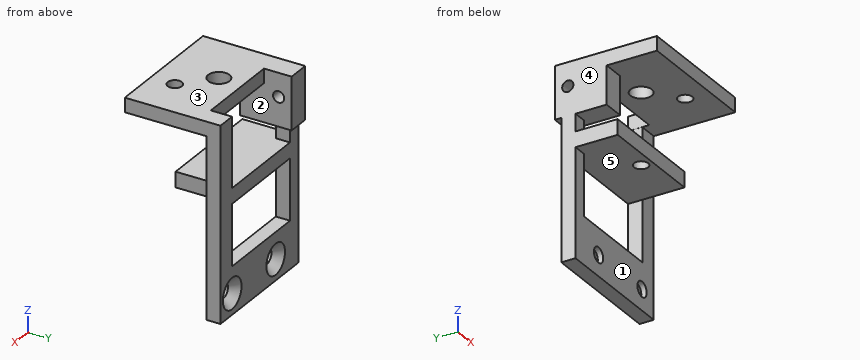
from build123d import *

# Parameters (mm, degrees)
SKETCH1_R                                        = 3.175
SKETCH1_R_2                                      = 4.762499999
BOSS_EXTRUDE1_DEPTH                              = 6.35
BOSS_EXTRUDE2_DEPTH                              = 23.368
SKETCH3_W                                        = 6.35
SKETCH3_H                                        = 78.34
SKETCH3_W_2                                      = 8.382
BOSS_EXTRUDE3_DEPTH                              = 6.35
CUT_EXTRUDE1_REACH                               = 104.101
SKETCH4_R                                        = 2.5
BOSS_EXTRUDE4_DEPTH                              = 6.35
CSK_FOR_1_4_FLAT_HEAD_MACHINE_SCREW1_D           = 6.7564
CSK_FOR_1_4_FLAT_HEAD_MACHINE_SCREW1_CSINK_D     = 13.6398
CSK_FOR_1_4_FLAT_HEAD_MACHINE_SCREW1_CSINK_ANGLE = 82
SKETCH8_W                                        = 48.768
SKETCH8_H                                        = 6.843039895
BOSS_EXTRUDE5_DEPTH                              = 25.146
CUT_EXTRUDE2_REACH                               = 68.059
SKETCH10_R                                       = 3.175


with BuildPart() as part:
    # Sketch1 → Boss-Extrude1 (new body)
    with BuildSketch(Plane.XY):
        Polygon((23.52260518, 29.069744957), (31.942128684, 29.069744957), (31.942128684, -13.602255043), (-25.207871316, -13.602255043), (-25.207871316, 8.844196721), (-25.207871316, 31.958196721), (-18.857871316, 31.958196721), (-15.310946905, 31.958196721), (-15.310946905, 22.656471706), (-15.310946905, 19.620299994), (23.52260518, 19.620299994), (23.52260518, 22.656471706), align=None)
        with Locations((12.892128684, -2.934255043)):
            Circle(SKETCH1_R, mode=Mode.SUBTRACT)
        with Locations((6.7e-08, 8.844196721)):
            Circle(SKETCH1_R_2, mode=Mode.SUBTRACT)
    extrude(amount=-BOSS_EXTRUDE1_DEPTH)

    # Sketch2 → Boss-Extrude2 (add)
    with BuildSketch(Plane.XY):
        Polygon((-15.310946905, 31.958196721), (-18.857871316, 31.958196721), (-25.207871316, 31.958196721), (-25.207871316, 8.844196721), (-18.857871316, 8.844196721), (-15.310946905, 8.844196721), (-15.310946905, 19.620299994), align=None)
    extrude(amount=-BOSS_EXTRUDE2_DEPTH)

    # Sketch3 → Boss-Extrude3 (add)
    with BuildSketch(Plane(origin=(0, 29.069744957, 0), x_dir=(1, 0, 0), z_dir=(0, 1, 0))):
        with Locations((-22.032871316, 39.17)):
            Rectangle(SKETCH3_W, SKETCH3_H)
        with Locations((27.751128684, 39.17)):
            Rectangle(SKETCH3_W_2, SKETCH3_H)
    extrude(amount=-BOSS_EXTRUDE3_DEPTH)

    # Sketch4 → Cut-Extrude1 (cut, up to next)
    with BuildSketch(Plane.ZY.offset(25.207871316), mode=Mode.PRIVATE) as cut_extrude1_sk1:
        with Locations(Location((-10.437499124, 26.162307082, 0), (0, 0, 270))):
            Circle(SKETCH4_R)
    cut_extrude1_tool1 = extrude(cut_extrude1_sk1.sketch, amount=-CUT_EXTRUDE1_REACH, mode=Mode.PRIVATE) & part.part
    add(cut_extrude1_tool1.solids().sort_by_distance((-25.207871, 26.162307, -10.437499))[0], mode=Mode.SUBTRACT)

    # Sketch5 → Boss-Extrude4 (add)
    with BuildSketch(Plane(origin=(0, 29.069744957, 0), x_dir=(1, 0, 0), z_dir=(0, 1, 0))):
        Polygon((-25.207871316, 78.34), (-25.207871316, 65.022649662), (31.942128684, 65.022649662), (31.942128684, 78.34), (31.942128684, 86.081334737), (-25.207871316, 86.081334737), align=None)
    extrude(amount=-BOSS_EXTRUDE4_DEPTH)

    # CSK for 1/4 Flat Head Machine Screw1 (through all)
    with Locations(Plane(origin=(0, 29.069744957, 0), x_dir=(1, 0, 0), z_dir=(0, 1, 0))):
        with Locations((-8.384740386, 76.819020678), (23.394249394, 76.819020678)):
            CounterSinkHole(CSK_FOR_1_4_FLAT_HEAD_MACHINE_SCREW1_D / 2, CSK_FOR_1_4_FLAT_HEAD_MACHINE_SCREW1_CSINK_D / 2, counter_sink_angle=CSK_FOR_1_4_FLAT_HEAD_MACHINE_SCREW1_CSINK_ANGLE)

    # Sketch8 → Boss-Extrude5 (add)
    with BuildSketch(Plane(origin=(0, 29.069744957, 0), x_dir=(1, 0, 0), z_dir=(0, 1, 0))):
        with Locations((-0.823871316, 34.471519947)):
            Rectangle(SKETCH8_W, SKETCH8_H)
    extrude(amount=-BOSS_EXTRUDE5_DEPTH)

    # Sketch10 → Cut-Extrude2 (cut, up to next)
    with BuildSketch(Plane(origin=(0, 0, -37.893039895), x_dir=(-1, 0, 0), z_dir=(0, 0, -1)), mode=Mode.PRIVATE) as cut_extrude2_sk1:
        with Locations((-6.7e-08, 8.844196721)):
            Circle(SKETCH10_R)
    cut_extrude2_tool1 = extrude(cut_extrude2_sk1.sketch, amount=-CUT_EXTRUDE2_REACH, mode=Mode.PRIVATE) & part.part
    add(cut_extrude2_tool1.solids().sort_by_distance((0, 8.844197, -37.89304))[0], mode=Mode.SUBTRACT)


solid = part.part
Could you check a few things on this model? Use its own coordinates, in mm. Face numbers are marked on the shaded views. A direction names the side the tool comes from. Round coordinates to 2 decimals unless told otherwise and drop trailing zeros. Loops run counter-clockwise (first coordinate to the right, second up) from the corner with the lowest first, then second, coordinate; pieces in that order, holes last. Notation, with made-up numbers: (53, 83.25) - (77, 83.25) arc R11 ccw to (77, 98.25) - close; hole circle Ø7 at (2, 19.25). An arc over 180 degrees is marked (long way). Write item = value, one per line.
1) On a 3-axis mill with a long thin cutter (end or side, diameter ignored), from which of +Z, -Z, +X, -X, +Y, -Y can I reach the whole of each face in a straight line? I mean the marked faces 1 and 2. Say none if no direction works.
Computed:
face_1 = -Z, +X, -Y
face_2 = +Y
2) Imagine slicing it at B-B (x = 0). Please give me the cut outline in (y, z).
Computed:
outline = (-13.6, -6.35) - (4.08, -6.35) - (4.08, 0) - (-13.6, 0) - close; (3.92, -37.89) - (5.67, -37.89) - (5.67, -31.05) - (3.92, -31.05) - close; (12.02, -37.89) - (29.07, -37.89) - (29.07, -31.05) - (12.02, -31.05) - close; (13.61, -6.35) - (19.62, -6.35) - (19.62, 0) - (13.61, 0) - close; (22.72, -86.08) - (29.07, -86.08) - (29.07, -65.02) - (22.72, -65.02) - close
3) If we mould it in two halves opening along X, with no side actions, what happens to the marked faces 3, 4 and 5? For each: pulls with the +X half, pulls with the -X half, needs draft (parallel to the pull), parting line crosses it, or undercut.
Computed:
face_3 = needs draft
face_4 = pulls with the -X half
face_5 = undercut
4) Imagine slicing it at D-D (x = 13). Please give me the cut outline in (y, z), and give its area (3 significant figures).
Computed:
outline = (-13.6, -6.35) - (-6.11, -6.35) - (-6.11, 0) - (-13.6, 0) - close; (0.24, -6.35) - (19.62, -6.35) - (19.62, 0) - (0.24, 0) - close; (3.92, -37.89) - (29.07, -37.89) - (29.07, -31.05) - (3.92, -31.05) - close; (22.72, -86.08) - (29.07, -86.08) - (29.07, -65.02) - (22.72, -65.02) - close
area = 476 mm2
5) I'm going to push flat-ended pins straight in: P1, Ø5, axis at x = 12.89, y = -2.93, coming from the +Z side; P2, Ø2, axis at x = 6.5, z = -71.5, coming from the +Y side; P3, Ø12, axis at x = -9.5, y = -6, coming from the -Z side; P4, Ø2, axis at x = 3, z = -34.5, coming from the -Y side. Where does each tip first touch, or does it pass through?
Computed:
P1 = through
P2 = 29.07
P3 = -6.35
P4 = 3.92
6) Imagine slicing it at C-C (y = -2). Please give me the cut outline in (x, z), and give its area (3 significant figures).
Computed:
outline = (-25.21, -6.35) - (9.86, -6.35) - (9.86, 0) - (-25.21, 0) - close; (15.93, -6.35) - (31.94, -6.35) - (31.94, 0) - (15.93, 0) - close
area = 324 mm2
7) Imagine slicing it at A-A (z = -60.5). Please give me the cut outline in (x, y).
Computed:
outline = (-25.21, 22.72) - (-18.86, 22.72) - (-18.86, 29.07) - (-25.21, 29.07) - close; (23.56, 22.72) - (31.94, 22.72) - (31.94, 29.07) - (23.56, 29.07) - close
8) I need wall thicknesses on line 1 along Z through (x, y) = (-10, 10); line 2 along Y through (x, z) = (0, -33.5); line 3 along X through (y, z) = (24, -38). Which ranges of each line are inside material? Lowest first, please. Write a range as from..to.
Computed:
line_1 = -37.89..-31.05, -6.35..0
line_2 = 3.92..5.67, 12.02..29.07
line_3 = -25.21..-18.86, 23.56..31.94
